Part model, mm, in its own coordinate system. A direction names the side the tool comes from. Round coordinates to 2 decimals unless told otherwise and drop trailing zeros. Loops run counter-clockwise (first coordinate to the right, second up) from the corner with the lowest first, then second, coordinate; pieces in that order, holes last. Notation, with made-up numbers: (-12, -31.75) -> (46, -31.75) arc R14 cw to (46, -20.75) -> close; hole circle Ø9 at (12, 80.25). An arc over 180 degrees is marked (long way). Answer as a JSON object with one key per item and string values. Group by question number.
from build123d import *

# Parameters (mm, degrees)
SKETCH1_W           = 330.2
SKETCH1_H           = 6.35
BOSS_EXTRUDE1_DEPTH = 25.4
BOSS_EXTRUDE2_DEPTH = 6.35
CUT_EXTRUDE1_DEPTH  = 168.16307158


with BuildPart() as part:
    # Sketch1 → Boss-Extrude1 (new body)
    with BuildSketch(Plane(origin=(0, 0, 0), x_dir=(1, 0, 0), z_dir=(0, 1, 0))):
        Rectangle(SKETCH1_W, SKETCH1_H)
    extrude(amount=BOSS_EXTRUDE1_DEPTH)

    # Sketch2 → Boss-Extrude2 (add)
    with BuildSketch(Plane.XZ):
        with BuildLine():
            Line((-133.35, 2.54), (-133.35, -2.54))
            ThreePointArc((-133.35, -2.54), (-135.89, 0), (-133.35, 2.54))
        make_face()
        with BuildLine():
            Line((0, 2.54), (0, -2.54))
            ThreePointArc((0, -2.54), (-2.54, 0), (0, 2.54))
        make_face()
        with BuildLine():
            Line((133.35, 2.54), (133.35, -2.54))
            ThreePointArc((133.35, -2.54), (130.81, 0), (133.35, 2.54))
        make_face()
    extrude(amount=BOSS_EXTRUDE2_DEPTH)

    # Sketch3 → Cut-Extrude1 (cut, through all)
    with BuildSketch(Plane.XY.offset(3.175)):
        with BuildLine():
            Line((-143.51, 38.1), (-143.51, 12.7))
            ThreePointArc((-143.51, 12.7), (-146.05, 10.16), (-148.59, 12.7))
            Line((-148.59, 12.7), (-148.59, 38.1))
            ThreePointArc((-148.59, 38.1), (-146.05, 40.64), (-143.51, 38.1))
        make_face()
        with BuildLine():
            Line((-106.68, 38.1), (-106.68, 12.7))
            ThreePointArc((-106.68, 12.7), (-109.22, 10.16), (-111.76, 12.7))
            Line((-111.76, 12.7), (-111.76, 38.1))
            ThreePointArc((-111.76, 38.1), (-109.22, 40.64), (-106.68, 38.1))
        make_face()
        with BuildLine():
            Line((-69.85, 38.1), (-69.85, 12.7))
            ThreePointArc((-69.85, 12.7), (-72.39, 10.16), (-74.93, 12.7))
            Line((-74.93, 12.7), (-74.93, 38.1))
            ThreePointArc((-74.93, 38.1), (-72.39, 40.64), (-69.85, 38.1))
        make_face()
        with BuildLine():
            Line((-33.02, 38.1), (-33.02, 12.7))
            ThreePointArc((-33.02, 12.7), (-35.56, 10.16), (-38.1, 12.7))
            Line((-38.1, 12.7), (-38.1, 38.1))
            ThreePointArc((-38.1, 38.1), (-35.56, 40.64), (-33.02, 38.1))
        make_face()
        with BuildLine():
            Line((3.81, 38.1), (3.81, 12.7))
            ThreePointArc((3.81, 12.7), (1.27, 10.16), (-1.27, 12.7))
            Line((-1.27, 12.7), (-1.27, 38.1))
            ThreePointArc((-1.27, 38.1), (1.27, 40.64), (3.81, 38.1))
        make_face()
        with BuildLine():
            Line((40.64, 38.1), (40.64, 12.7))
            ThreePointArc((40.64, 12.7), (38.1, 10.16), (35.56, 12.7))
            Line((35.56, 12.7), (35.56, 38.1))
            ThreePointArc((35.56, 38.1), (38.1, 40.64), (40.64, 38.1))
        make_face()
        with BuildLine():
            Line((77.47, 38.1), (77.47, 12.7))
            ThreePointArc((77.47, 12.7), (74.93, 10.16), (72.39, 12.7))
            Line((72.39, 12.7), (72.39, 38.1))
            ThreePointArc((72.39, 38.1), (74.93, 40.64), (77.47, 38.1))
        make_face()
        with BuildLine():
            Line((114.3, 38.1), (114.3, 12.7))
            ThreePointArc((114.3, 12.7), (111.76, 10.16), (109.22, 12.7))
            Line((109.22, 12.7), (109.22, 38.1))
            ThreePointArc((109.22, 38.1), (111.76, 40.64), (114.3, 38.1))
        make_face()
        with BuildLine():
            Line((151.13, 38.1), (151.13, 12.7))
            ThreePointArc((151.13, 12.7), (148.59, 10.16), (146.05, 12.7))
            Line((146.05, 12.7), (146.05, 38.1))
            ThreePointArc((146.05, 38.1), (148.59, 40.64), (151.13, 38.1))
        make_face()
    extrude(amount=-CUT_EXTRUDE1_DEPTH, mode=Mode.SUBTRACT)


solid = part.part
Item 1: Which spindle directions (+Z, -Z, +X, -X, +Y, -Y) get a long thin tool onto all of the face, cutting with end or side? Do faces 1 (the face through (0, -3, 0)), 2 (the face through (-157, 25.4, 0)), 3 (the face through (-2, 13, -3.175)), 4 (the face through (-135.89, -3.13, -0.06)), 5 (the face through (-143.51, 19, 0)). Say none if no direction does.
Item 2: Band-saw the part on C-C, the plane x = 106. List the corners of the cut face in (y, z) (3 decimals), plus the area to 3 significant figures.
Item 3: Band-saw the part on B-B, the plane y = 22.5. Count the separate pieces of the cut face and the enclosed holes in it, plus the area to 3 significant figures.
Item 4: Drill centre lines: line 1 (Y direction, x = -117.5, z = -2.5); line 2 (Y direction, x = 73, z = 0.75). Where is each one in solid material? Low to high.
Item 5: Band-saw the part on A-A, the plane y = -3.5. List the corners of the cut face in (x, z), plus the area to 3 significant figures.
Item 6: Drop flat-ended pins along their axis: pin 1 Ø2 at (y, z) = (-3, 0) entering from -X; pin 2 Ø1.5 at (x, z) = (-95, 1) entering from -Y. Give the stop position or say it passes through.
Item 7: Two-plate mould, pull along X, no slides. Class faces 6 (the face through (130, 25.4, 0)), 7 (the face through (72.39, 19, 0)), 8 (the face through (38.16, 10.16, 0.04)), 9 (the face through (133.35, -3, 0)): pulls with the +X half, pulls with the -X half, needs draft (parallel to the pull), parting line crosses it, or undercut.
Entries:
{
 "1": {"face 1": "+Z, -Z, -Y", "face 2": "+Z, -Z, +X, -X, +Y", "face 3": "-Z, +X, -X, +Y, -Y", "face 4": "-X, -Y", "face 5": "+Z, -Z, +Y"},
 "2": {"outline": "(0, -3.175) -> (25.4, -3.175) -> (25.4, 3.175) -> (0, 3.175) -> close", "area": "161 mm²"},
 "3": {"separate pieces": "10", "enclosed holes": "0", "area": "1,810 mm²"},
 "4": {"line 1": "0 to 25.4", "line 2": "0 to 11.05"},
 "5": {"outline": "(-133.35, -2.54) -> (-133.35, 2.54) arc R2.54 ccw to start; (0, -2.54) -> (0, 2.54) arc R2.54 ccw to start; (133.35, -2.54) -> (133.35, 2.54) arc R2.54 ccw to start", "area": "30.4 mm²"},
 "6": {"pin 1": "x = -135.89", "pin 2": "y = 0"},
 "7": {"face 6": "needs draft", "face 7": "undercut", "face 8": "undercut", "face 9": "pulls with the +X half"}
}
